```python
from build123d import *

# Parameters (mm, degrees)
SKETCH051_R        = 5.75
SKETCH051_R_2      = 3.75
PAD012002_DEPTH    = 2.25
PAD012003_DEPTH    = 3.5
POCKET003052_DEPTH = 2.65
SKETCH054_R        = 3.75
SKETCH054_R_2      = 0.75
POCKET003053_DEPTH = 5
SKETCH055_R        = 1.25
PAD012004_DEPTH    = 2


with BuildPart() as part:
    # Sketch051 → Pad012002 (new body)
    with BuildSketch(Plane.XY):
        Circle(SKETCH051_R)
        Circle(SKETCH051_R_2, mode=Mode.SUBTRACT)
    extrude(amount=PAD012002_DEPTH)

    # Sketch053 (on Face4 of Pad012002) → Pad012003 (join)
    with BuildSketch(Plane.XY.offset(2.25)):
        with BuildLine():
            Line((0, 5.714965), (-20.5, 5.714965))
            Line((-20.5, 5.714965), (-20.5, -5.714965))
            Line((0, -5.714965), (-20.5, -5.714965))
            ThreePointArc((0, -5.714965), (5.714965, 0), (0, 5.714965))
        make_face()
    extrude(amount=PAD012003_DEPTH)

    # Sketch052 (on Face11 of Pad012003) → Pocket003052 (cut)
    with BuildSketch(Plane.XY.offset(5.75)):
        with BuildLine():
            Line((-1.25, 3.535534), (-16.999999, 1.742953))
            ThreePointArc((-16.999999, 1.742953), (-18.232454, 1.232454), (-18.742953, 0))
            ThreePointArc((-18.742953, 0), (-18.232454, -1.232454), (-16.999999, -1.742953))
            Line((-1.25, -3.535534), (-16.999999, -1.742953))
            ThreePointArc((-1.25, -3.535534), (2.165064, -3.061862), (3.75, 0))
            ThreePointArc((3.75, 0), (2.165064, 3.061862), (-1.25, 3.535534))
        make_face()
    extrude(amount=-POCKET003052_DEPTH, mode=Mode.SUBTRACT)

    # Sketch054 (on Face16 of Pocket003052) → Pocket003053 (cut)
    with BuildSketch(Plane.XY.offset(3.1)):
        Circle(SKETCH054_R)
        with Locations((-14.5, 0)):
            Circle(SKETCH054_R_2)
        with Locations((-12.5, 0)):
            Circle(SKETCH054_R_2)
        with Locations((-10.5, 0)):
            Circle(SKETCH054_R_2)
        with Locations((-8.5, 0)):
            Circle(SKETCH054_R_2)
        with Locations((-6.5, 0)):
            Circle(SKETCH054_R_2)
    extrude(amount=-POCKET003053_DEPTH, mode=Mode.SUBTRACT)

    # Sketch055 (on Face2 of Pocket003053) → Pad012004 (join)
    with BuildSketch(Plane.XZ.offset(5.714965)):
        with BuildLine():
            Line((-20.5, 2.25), (0, 2.25))
            ThreePointArc((0, 2.25), (2.563672, 13.869245), (-4.309476, 23.582077))
            Line((-24.748606, 35.382614), (-4.309476, 23.582077))
            ThreePointArc((-24.748606, 35.382614), (-30.040757, 36.079339), (-34.275532, 32.829882))
            Line((-36.844536, 28.380237), (-34.275532, 32.829882))
            ThreePointArc((-36.844536, 28.380237), (-37.534628, 23.138468), (-34.316106, 18.944009))
            Line((-34.316106, 18.944009), (-19.282618, 10.264421))
            ThreePointArc((-20.5, 5.75), (-18.301189, 7.578411), (-19.282618, 10.264421))
            Line((-20.5, 5.75), (-20.5, 2.25))
        make_face()
        with Locations((-31.113487, 28.115616)):
            Circle(SKETCH055_R, mode=Mode.SUBTRACT)
        with Locations((-7.608902, 14.5)):
            Circle(SKETCH055_R, mode=Mode.SUBTRACT)
        Polygon((-32.740181, 21.49825), (-26.230181, 32.773901), (-5.913225, 21.043901), (-12.423225, 9.76825), align=None, mode=Mode.SUBTRACT)
    extrude(amount=-PAD012004_DEPTH)


with BuildPart() as part_1:
    # Body010 placement: moved
    add(part.part.moved(Location((0, 0, 44))))


solid = part_1.part
```
The model under review builds one solid part; all positions refer to its coordinate system, in mm. A direction names the side the tool comes from. Round coordinates to 2 decimals unless told otherwise and drop trailing zeros. Loops run counter-clockwise (first coordinate to the right, second up) from the corner with the lowest first, then second, coordinate; pieces in that order, holes last. Notation, with made-up numbers: M 16.5,2.25 L 50.5,2.25 A8 ccw 50.5,7.25 Z; hole C 55.25,35.25 d5. An arc over 180 degrees is marked long. Answer as a JSON object with one key per item and string values.
(1) Tool access review of faces 4 (the cylindrical face through (-0.75, 5.7, 45.11)), 5 (the flat face through (-10, 5.715, 48)), 6 (the flat face through (-9.12, -4.73, 59.49)), 7 (the flat face through (-9.015, 2.652, 48.444)), 8 (the cylindrical face through (-7.25, 0.03, 46.68)): name each direction out of +Z, -Z, +X, -X, +Y, -Y from which nothing blocks a thin tool from reaching the whole face with its end or side.
Resolved:
{"face 4": "-Z", "face 5": "+Z, -Z, +X, -X, +Y", "face 6": "+Y, -Y", "face 7": "+Z", "face 8": "+Z, -Z"}
(2) Take a section at D-D on z = 58.5. Give the boundary of the cut face in (x, y), and give its area (3 significant figures).
Resolved:
{"outline": "M -26.62,-5.71 L -20.62,-5.71 L -20.62,-3.71 L -26.62,-3.71 Z; M -9.69,-5.71 L -8.86,-5.71 L -8.86,-3.71 L -9.69,-3.71 Z; M -6.36,-5.71 L 2.42,-5.71 L 2.42,-3.71 L -6.36,-3.71 Z", "area": "31.2 mm²"}
(3) Take a section at C-C on z = 75. Give the boundary of the cut face in (x, y).
Resolved:
{"outline": "M -35.33,-5.71 L -27.25,-5.71 L -27.25,-3.71 L -35.33,-3.71 Z; M -23.16,-5.71 L -17.16,-5.71 L -17.16,-3.71 L -23.16,-3.71 Z"}
(4) Draft analysis for pull direction Z (two halves, no side actions). For faces 1 (the flat face through (-35.58, -4.73, 74.57)), 2 (the cylindrical face through (5.714, -0.126, 47.976)), 3 (the flat face through (4, 0, 44)), state which applies: released by +Z, released by -Z, zero draft, split by the parting line, or undercut.
Resolved:
{"face 1": "released by +Z", "face 2": "undercut", "face 3": "released by -Z"}
(5) To check wall thickness, follow line 1 along Y through (x, z) = (-14.5, 46.6); line 2 along Y through (x, z) = (0, 45.85); line 3 along Y through (x, z) = (-19, 47). State the ranges of each line that lie inside material, in increasing order.
Resolved:
{"line 1": "-5.71 to -0.75, 0.75 to 5.71", "line 2": "-5.75 to -3.75, 3.75 to 5.75", "line 3": "-5.71 to 5.71"}
(6) Clearance check with flat-ended pins moving along their axes: P1, Ø3, axis at x = -7.61, z = 58.5, coming from the +Y side; P2, Ø2.5, axis at x = -14.5, y = 0, coming from the +Z side; P3, Ø6, axis at x = -13.5, z = 50.5, coming from the +Y side. State where each tip first meets the part, or that it passes through.
Resolved:
{"P1": "y = -3.71", "P2": "z = 47.1", "P3": "y = 5.71"}
(7) Take a section at A-A on x = -14.5. Give the boundary of the cut face in (y, z), and give its area (3 significant figures).
Resolved:
{"outline": "M -5.71,46.25 L -0.75,46.25 L -0.75,47.1 L -2.03,47.1 L -2.03,49.75 L -3.71,49.75 L -3.71,54.97 L -5.71,54.97 Z; M -5.71,70 L -3.71,70 L -3.71,73.47 L -5.71,73.47 Z; M 0.75,46.25 L 5.71,46.25 L 5.71,49.75 L 2.03,49.75 L 2.03,47.1 L 0.75,47.1 Z", "area": "45.3 mm²"}
